Source: CAD feature listing. Evaluate the final solid. Frame: model axes, mm. Face numbers are marked on the shaded views. Give positions to 0.01 mm unless a question says otherwise; leave off trailing zeros. Loops run counter-clockwise (first coordinate to the right, second up) from the corner with the lowest first, then second, coordinate; pieces in that order, holes last. Notation, with made-up numbers: M -31.75,24.25 L 26.25,24.25 A20 ccw 26.25,50.25 Z; hole C -29.75,-16 d5. An arc over 180 degrees is marked long. Write item = value, one per line.
from build123d import *

# Parameters (mm, degrees)
SKETCH1_R               = 5
BOSS_EXTRUDE1_DEPTH     = 4
SKETCH2_OUTSIDE_W       = 56.08
SKETCH2_OUTSIDE_H       = 59.128
SKETCH2_OUTSIDE_R       = 10
CUT_EXTRUDE1_DEPTH      = 8
CUT_EXTRUDE1_DRAFT      = -60
MIRROR1_COPY_1_SKETCH_W = 56.08
MIRROR1_COPY_1_SKETCH_H = 59.128
MIRROR1_COPY_1_SKETCH_R = 10
MIRROR1_COPY_1_DEPTH    = 8
MIRROR1_COPY_1_DRAFT    = -60


with BuildPart() as part:
    # Sketch1 → Boss-Extrude1 (new, symmetric)
    with BuildSketch(Plane.XY):
        Polygon((10.023495122, -5.732615361), (9.976338094, 5.81429373), (-0.047157028, 11.546909091), (-10.023495122, 5.732615361), (-9.976338094, -5.81429373), (0.047157028, -11.546909091), align=None)
        Circle(SKETCH1_R, mode=Mode.SUBTRACT)
    extrude(amount=BOSS_EXTRUDE1_DEPTH, both=True)


with BuildPart() as cut_extrude1_tool:
    # Sketch2 outside → Cut-Extrude1 (with draft: the straight prism first)
    with BuildSketch(Plane(origin=(0, 0, -4), x_dir=(-1, 0, 0), z_dir=(0, 0, -1))):
        Rectangle(SKETCH2_OUTSIDE_W, SKETCH2_OUTSIDE_H)
        Circle(SKETCH2_OUTSIDE_R, mode=Mode.SUBTRACT)
    extrude(amount=-CUT_EXTRUDE1_DEPTH)
    # Cut-Extrude1: the draft: its side faces are tilted about the plane it starts from
    cut_extrude1_sides = [cut_extrude1_tool.faces().sort_by_distance(p)[0] for p in [
        (0, -29.564, 0),
        (-28.04, 0, 0),
        (0, 29.564, 0),
        (28.04, 0, 0),
        (10, 0, 0),
    ]]
    draft(cut_extrude1_sides, Plane(origin=(0, 0, -4), x_dir=(-1, 0, 0), z_dir=(0, 0, -1)), CUT_EXTRUDE1_DRAFT)


with BuildPart() as part_1:
    add(part.part)

    # Cut-Extrude1: cut by cut_extrude1_tool
    add(cut_extrude1_tool.part, mode=Mode.SUBTRACT)


with BuildPart() as mirror1_copy_1_tool:
    # Mirror1 copy 1 sketch → Mirror1 copy 1 (with draft: the straight prism first)
    with BuildSketch(Plane(origin=(0, 0, 4), x_dir=(-1, 0, 0), z_dir=(0, 0, 1))):
        Rectangle(MIRROR1_COPY_1_SKETCH_W, MIRROR1_COPY_1_SKETCH_H)
        Circle(MIRROR1_COPY_1_SKETCH_R, mode=Mode.SUBTRACT)
    extrude(amount=-MIRROR1_COPY_1_DEPTH)
    # Mirror1 copy 1: the draft: its side faces are tilted about the plane it starts from
    mirror1_copy_1_sides = [mirror1_copy_1_tool.faces().sort_by_distance(p)[0] for p in [
        (0, -29.564, 0),
        (-28.04, 0, 0),
        (0, 29.564, 0),
        (28.04, 0, 0),
        (10, 0, 0),
    ]]
    draft(mirror1_copy_1_sides, Plane(origin=(0, 0, 4), x_dir=(-1, 0, 0), z_dir=(0, 0, 1)), MIRROR1_COPY_1_DRAFT)


with BuildPart() as part_2:
    add(part_1.part)

    # Mirror1 copy 1: cut by mirror1_copy_1_tool
    add(mirror1_copy_1_tool.part, mode=Mode.SUBTRACT)


solid = part_2.part
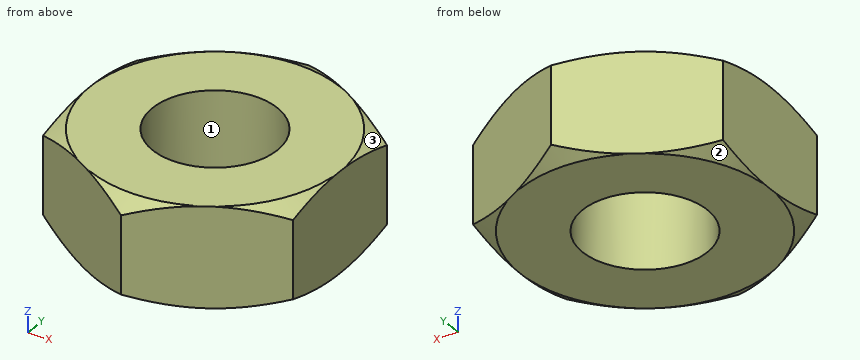
1. First-contact query: pin 1 Ø4 at (x, z) = (3.5, 2) entering from -Y; pin 2 Ø1 at (y, z) = (-8, -3) entering from -X; pin 3 Ø10 at (x, y) = (-2, -4) entering from +Z; pin 4 Ø1.5 at (x, z) = (8, -1.5) entering from -Y. Flat tips, straight axial feed; report the tip coordinate or a pass-through.
Derived:
pin_1 = -10.7
pin_2 = -7.03
pin_3 = 4
pin_4 = -7.35
2. Pull-direction query (X, two-part tool) for the marked faces 1, 2 and 3; classes: +X half, -X half, draft (parallel to the pull), parting line (faces both ways), or undercut.
Derived:
face_1 = undercut
face_2 = -X half
face_3 = +X half
3. Material intervals for probe 1 along X at (y, z) = (-3, 1.75); probe 2 along Y at (x, z) = (0, 1.5); probe 3 along X at (y, z) = (5.5, -1.5), sorted ascending. Write a range as from..to.
Derived:
probe_1 = -9.99..-4, 4..10.01
probe_2 = -11.52..-5, 5..11.52
probe_3 = -10.02..9.98
4. Cut plane A-A, the plane z = -1.5. Return the cut outline in (x, y), then the cut area to 3 significant figures.
Derived:
outline = M -10.02,5.73 L -9.98,-5.81 L 0.05,-11.55 L 10.02,-5.73 L 9.98,5.81 L -0.05,11.55 Z; hole C 0,0 d10
area = 268 mm²
